```python
from build123d import *

# Parameters (mm, degrees)
F0_W     = 68.38
F0_H     = 53.52
F1_DEPTH = 19.18835
F2_W     = 9.33
F2_H     = 9.33
F3_DEPTH = 10.86
F4_R     = 20
F5_R     = 20
F7_W     = 25
F7_H     = 30
F7_W_2   = 6.7
F7_H_2   = 6.7
F8_DEPTH = 29.55052


with BuildPart() as f1:
    # F0 (on Top) → F1 (new body)
    with BuildSketch(Plane.XY):
        Rectangle(F0_W, F0_H)
    extrude(amount=F1_DEPTH)

    # F2 (on face) → F3 (join)
    with BuildSketch(Plane(origin=(-34.19, 0, 0), x_dir=(0, -1, 0), z_dir=(-1, 0, 0))):
        with Locations((-22.095, 14.52335)):
            Rectangle(F2_W, F2_H)
    extrude(amount=F3_DEPTH)

    # F4
    f4_edges = [f1.edges().sort_by_distance(p)[0] for p in [
        (34.19, -26.76, 9.594175),
    ]]
    fillet(f4_edges, radius=F4_R)

    # F5
    f5_edges = [f1.edges().sort_by_distance(p)[0] for p in [
        (-34.19, -26.76, 9.594175),
    ]]
    fillet(f5_edges, radius=F5_R)

    # F7 (on face) → F8 (cut)
    with BuildSketch(Plane.XY):
        with Locations((-11.69, 1.76)):
            Rectangle(F7_W, F7_H)
        with Locations((13.863151, 13.41)):
            Rectangle(F7_W_2, F7_H_2)
        with Locations((13.863151, 1.91)):
            Rectangle(F7_W_2, F7_H_2)
        with Locations((13.863151, -9.59)):
            Rectangle(F7_W_2, F7_H_2)
    extrude(amount=F8_DEPTH, mode=Mode.SUBTRACT)


solid = f1.part
```
Part model, mm, in its own coordinate system. A direction names the side the tool comes from. Round coordinates to 2 decimals unless told otherwise and drop trailing zeros. Loops run counter-clockwise (first coordinate to the right, second up) from the corner with the lowest first, then second, coordinate; pieces in that order, holes last.
Item 1: Drop flat-ended pins along their axis: P1, Ø3.5, axis at y = 2.5, z = 10, coming from the -X side; P2, Ø7.5, axis at x = -42, z = 12.5, coming from the -Y side; P3, Ø2, axis at y = -11, z = 9, coming from the -X side; P4, Ø8, axis at x = 17, y = 7, coming from the -Z side. Give the stop position or say it passes through.
Item 2: Cut at D-D, the plane y = -11. Give the cut face in (x, z), then the cut area to 3 significant figures.
Item 3: Cut at A-A, the plane y = 9. Give the cut face in (x, z).
Item 4: 3-axis set-ups, long thin cutter, end or side, ignore diameter. For faces 1 (the face through (-12, 16.76, 9)), 2 (the face through (-40, 22, 9.858)), 3 (the face through (-40, 17.43, 14)): which of +Z, -Z, +X, -X, +Y, -Y reach the whole face in a straight line?
Item 5: Cut at B-B, the plane z = 13.75. Give the cut face in (x, y), then the cut area to 3 significant figures.
Item 6: Drill centre lines: line 1 (X direction, y = 16.5, z = 5); line 2 (X direction, y = 9, z = 7.75); line 3 (Y direction, x = -2.5, z = 4.75). Where is each one in solid material? Low to high.
Item 7: Cut at C-C, the plane x = -16.5. Give the cut face in (y, z).
Item 8: Mould opens along X. For faces 4 (the face through (10.513, 13, 9)), 5 (the face through (-45.05, 22, 15)), 6 (the face through (0, -26.76, 9)) say: +X half, -X half, draft (parallel to the pull), parting line (faces both ways), or undercut.
A:
1. P1: stops at x = -34.19
1. P2: stops at y = 17.43
1. P3: stops at x = -33.93
1. P4: stops at z = 0
2. outline: (-33.74, 0) - (-24.19, 0) - (-24.19, 19.19) - (-33.74, 19.19) - close; (0.81, 0) - (10.51, 0) - (10.51, 19.19) - (0.81, 19.19) - close; (17.21, 0) - (33.74, 0) - (33.74, 19.19) - (17.21, 19.19) - close
2. area: 686 mm2
3. outline: (-34.19, 0) - (-24.19, 0) - (-24.19, 19.19) - (-34.19, 19.19) - close; (0.81, 0) - (34.19, 0) - (34.19, 19.19) - (0.81, 19.19) - close
4. face 1: +Z, -Z
4. face 2: -Z, -X, +Y, -Y
4. face 3: +Z, -Z, -X, -Y
5. outline: (-45.05, 17.43) - (-34.19, 17.43) - (-34.19, -6.76) arc R20 ccw to (-14.19, -26.76) - (14.19, -26.76) arc R20 ccw to (34.19, -6.76) - (34.19, 26.76) - (-45.05, 26.76) - close; hole (-24.19, -13.24) - (0.81, -13.24) - (0.81, 16.76) - (-24.19, 16.76) - close; hole (10.51, -12.94) - (17.21, -12.94) - (17.21, -6.24) - (10.51, -6.24) - close; hole (10.51, -1.44) - (17.21, -1.44) - (17.21, 5.26) - (10.51, 5.26) - close; hole (10.51, 10.06) - (17.21, 10.06) - (17.21, 16.76) - (10.51, 16.76) - close
5. area: 2,700 mm2
6. line 1: x = -34.19 to -24.19, 0.81 to 10.51, 17.21 to 34.19
6. line 2: x = -34.19 to -24.19, 0.81 to 34.19
6. line 3: y = -26.76 to -13.24, 16.76 to 26.76
7. outline: (-26.63, 0) - (-13.24, 0) - (-13.24, 19.19) - (-26.63, 19.19) - close; (16.76, 0) - (26.76, 0) - (26.76, 19.19) - (16.76, 19.19) - close
8. face 4: undercut
8. face 5: -X half
8. face 6: draft
